Autodesk Inventor part; units mm, degrees
ref_plane "YZ Plane" through (0, 0, 0) normal (1, 0, 0) x (0, 1, 0)
ref_plane "XZ Plane" through (0, 0, 0) normal (0, 1, 0) x (-1, 0, 0)
ref_plane "XY Plane" through (0, 0, 0) normal (0, 0, 1) x (1, 0, 0)
sketch "Skizze1" plane through (0, 0, 0) normal (0, 0, 1) x (1, 0, 0)
  line L0 (-17.073, 0) -> (17.073, 0)
  line L1 (0, -17.073) -> (0, 17.073)
  circle A0 centre (0, 0) radius 12.195
  dimension "d0" = 24.39
extrude "Extrusion1" add sketch "Skizze1" along normal mid plane 10.23
sketch "Skizze2" plane through (0, 0, 5.115) normal (0, 0, 1) x (1, 0, 0)
  circle A0 centre (0, 0) radius 12.195
  circle A1 centre (0, 0) radius 8
  dimension "d3" = 16
extrude "Extrusion2" cut sketch "Skizze2" against normal blind 4.615 contours A1
chamfer "Fase1" distance 0.2 angle 45 1 edges at (-8, 0, 5.115)
mirror "Spiegeln1" about plane through (0, 0, 0) normal (0, 0, 1) of "Extrusion2"
chamfer "Fase2" distance 0.2 angle 45 1 edges at (-8, 0, -5.115)
sketch "Skizze3" plane through (0, 0, 0.5) normal (0, 0, 1) x (1, 0, 0)
  circle A0 centre (0, 0) radius 8
  circle A1 centre (0, 0) radius 6.945
  dimension "d12" = 13.89
extrude "Extrusion3" cut sketch "Skizze3" against normal blind 1 contours A1
sketch "Skizze4" plane through (0, 0, 0) normal (0, 1, 0) x (-1, 0, 0)
  line L0 (17.073, 0) -> (-17.073, 0)
  line L1 (0, -7.161) -> (0, 7.161)
  line L2 (-12.195, -5.115) -> (12.195, -5.115)
  line L3 (12.195, 5.115) -> (-12.195, 5.115)
  line L4 (-12.195, -5.115) -> (-12.195, 5.115)
  line L5 (-12.195, -5.115) -> (12.195, -5.115)
  line L6 (-9.7834, -5.115) -> (-12.195, -2.69)
  line L7 (-12.195, -2.69) -> (-9.77, -0.2784)
  line L8 (-9.77, -0.2784) -> (-9.375, -0.2784)
  line L9 (-9.375, -0.2784) -> (-9.375, 0.2784)
  line L10 (-9.375, 0.2784) -> (-9.7834, 0.2784)
  line L11 (-9.7834, 0.2784) -> (-12.195, 2.7034)
  line L12 (-12.195, 2.7034) -> (-9.77, 5.115)
  line L13 (12.195, 5.115) -> (-12.195, 5.115)
  point P0 (0, 0)
  dimension "d15" = 3.42
  dimension "d17" = 9.375
  dimension "d18" = 9.77
revolve "Umdrehung1" cut sketch "Skizze4" angle 360 about axis through (0, 0, -10) along (0, 0, 1) contours L9 L8 L7 L4 L0 | L0 L4 L11 L10 L9 | L2 L4 L6 | L12 L4 L3
properties part number "Delrin_Dual_V"
Geometry: final body of the model. Coordinates: model frame, mm. A direction names the side the tool comes from. Round coordinates to 2 decimals unless told otherwise and drop trailing zeros. Loops run counter-clockwise (first coordinate to the right, second up) from the corner with the lowest first, then second, coordinate; pieces in that order, holes last.
Q1. Material intervals for L1, parallel to Y at x = -6.5, z = 2.5; L2, parallel to Y at x = 0, z = 2.9; L3, parallel to Z at x = 2.25, y = -9.5 (3 decimals), sorted ascending.
Q2. Pull-direction query (Y, two-part tool) for faces 1 (the conical face through (4.58, 8.8, -0.43)), 2 (the flat face through (-7, -5, -5.115)), 3 (the flat face through (-2, 7, 0.5)); classes: released by +Y, released by -Y, zero draft, split by the parting line, or undercut.
Q3. Section C-C on z = 1.25. Return loops of the section in (x, y).
Q4. Access query for faces 4 (the flat face through (2, 7, -0.5)), 5 (the cylindrical face through (-1.51, -6.78, 0.01)), 6 (the cylindrical face through (-1.22, 9.295, 0.004)), 7 (the cylindrical face through (-1.73, -7.81, 2.74)). Directions: +Z, -Z, +X, -X, +Y, -Y. A direction counts if a zero-diameter tool reaches every point of the face in a straight line with its end or side. Return the directions, or none.
Q5. Section D-D on z = 4. Return loops of the section in (x, y), plus the area to 3 significant figures.
Q6. Pin query (flat end, axial travel): P1, Ø4, axis at x = -3, z = -2.5, coming from the -Y side; P2, Ø1.5, axis at y = -2.5, z = 4, coming from the +X side; P3, Ø4, axis at x = -7, z = -1, coming from the -Y side. Return the tip coordinate at first contact, or that it passes through.
Evaluation:
1. L1: y = -10.08 to -4.66, 4.66 to 10.08
1. L2: y = -12 to -8, 8 to 12
1. L3: z = -5.115 to -0.278, 0.278 to 5.115
2. face 1: split by the parting line
2. face 2: zero draft
2. face 3: undercut
3. outline: circle Ø21.5 at (0, 0); hole circle Ø16 at (0, 0)
4. face 4: -Z
4. face 5: +Z, -Z
4. face 6: none
4. face 7: +Z
5. outline: circle Ø21.78 at (0, 0); hole circle Ø16 at (0, 0)
5. area: 172 mm2
6. P1: stops at y = -12.15
6. P2: stops at x = 11.39
6. P3: stops at y = -10.66
